Can you work these out from the model? Positions are in its coordinate system, mm. A direction names the side the tool comes from. Coordinates: 2 decimals unless noted, no trailing zeros. Order: outer loops, then holes, each group sorted by start corner. A loop starts at its lowest first (then second) coordinate and runs counter-clockwise, first axis right, second up. Notation, with made-up numbers: (-2, 42) -> (3, 42) arc R20 cw to (3, 51) -> close; hole circle Ø1 at (59.5, 17). An arc over 180 degrees is marked (long way). Answer in a Markdown table with one row per item. Add a question column.
1. Imagine slicing it at D-D on y = -6. Write out the boundary of the cut face in (x, z).
2. On a 3-axis mill with a long thin cutter (end or side, diameter ignored), from which of +Z, -Z, +X, -X, +Y, -Y can I reach the whole of each face in a straight line? I mean faces 1 (the face through (2, -2, 2.5)), 2 (the face through (-5, 0, 40)), 3 (the face through (0, 6, 5)). Say none if no direction works.
3. Imagine slicing it at A-A on y = 0. Write out the boundary of the cut face in (x, z).
4. Imagine slicing it at C-C on x = 0. Write out the boundary of the cut face in (y, z), plus the area to 3 significant figures.
5. We'd pull the mould along Y, two halves only. Please class faces 4 (the face through (-0.29, 2.23, 1.23)), 5 (the face through (5, 0, 40)), 6 (the face through (-3.746, 0.165, 21.512)): pulls with the +Y half, pulls with the -Y half, needs draft (parallel to the pull), parting line crosses it, or undercut.
6. Will these pins go through, and if not, where does the flat tip stop? pin 1 (2 mm diameter, centred on y = 7, z = 18.5, fed in from -X); pin 2 (2 mm diameter, centred on x = -2.5, z = 23, fed in from -Y); pin 3 (1.5 mm diameter, centred on y = -6, z = 10.5, fed in from -X).
7. Imagine slicing it at B-B on z = 17.5. Write out the boundary of the cut face in (x, y), plus the area to 3 significant figures.
8. If I drill on line 1 along X through (y, z) = (0, 10); line 2 along Y through (x, z) = (0, 1.25), over which ranges is the centre line in solid material (lowest first)? Write a range as [from, to].
from build123d import *
from build123d.topology import SkipClean

# Parameters (mm, degrees)
CROQUIS1_R              = 10
CROQUIS1_R_2            = 2.25
SALIENTE_EXTRUIR1_DEPTH = 5
SALIENTE_EXTRUIR2_DEPTH = 35
CROQUIS3_R              = 1.5
CORTAR_EXTRUIR1_DEPTH   = 20
CROQUIS4_R              = 3.75
CORTAR_EXTRUIR2_DEPTH   = 2.5
CORTAR_EXTRUIR4_START   = 49
CROQUIS6_R              = 3.75
CORTAR_EXTRUIR4_DEPTH   = 49


with BuildPart() as part:
    # Croquis1 → Saliente-Extruir1 (new body)
    with BuildSketch(Plane.XY):
        Circle(CROQUIS1_R)
        Circle(CROQUIS1_R_2, mode=Mode.SUBTRACT)
    extrude(amount=SALIENTE_EXTRUIR1_DEPTH)

    # Croquis2 → Saliente-Extruir2 (add)
    with SkipClean():  # the faces are left unmerged after this step: merging them gives an invalid solid
        with BuildSketch(Plane.XY.offset(5)):
            with BuildLine():
                Line((-2.5, -9.682458366), (-2.5, 9.682458366))
                ThreePointArc((-2.5, 9.682458366), (-10, 0), (-2.5, -9.682458366))
            make_face()
            with BuildLine():
                Line((2.5, -9.682458366), (2.5, 9.682458366))
                ThreePointArc((2.5, 9.682458366), (10, 0), (2.5, -9.682458366))
            make_face()
        extrude(amount=SALIENTE_EXTRUIR2_DEPTH)
    add(part.part.scale(1), mode=Mode.REPLACE)  # the faces are merged on a copy

    # Croquis3 → Cortar-Extruir1 (cut, symmetric)
    with BuildSketch(Plane.ZY.offset(-2.5)):
        with Locations((35, 0)):
            Circle(CROQUIS3_R)
    extrude(amount=CORTAR_EXTRUIR1_DEPTH, both=True, mode=Mode.SUBTRACT)

    # Croquis4 → Cortar-Extruir2 (cut)
    with BuildSketch(Plane.XY.offset(5)):
        Circle(CROQUIS4_R)
    extrude(amount=-CORTAR_EXTRUIR2_DEPTH, mode=Mode.SUBTRACT)

    # Croquis6 → Cortar-Extruir4 (cut)
    with SkipClean():  # the faces are left unmerged after this step: merging them gives an invalid solid
        with BuildSketch(Plane.XY.offset(2.5).offset(CORTAR_EXTRUIR4_START)):
            Circle(CROQUIS6_R)
        extrude(amount=-CORTAR_EXTRUIR4_DEPTH, mode=Mode.SUBTRACT)


solid = part.part
Answers follow:
| question | item | result |
|---|---|---|
| 1 | outline | (-8, 0) -> (8, 0) -> (8, 40) -> (2.5, 40) -> (2.5, 5) -> (-2.5, 5) -> (-2.5, 40) -> (-8, 40) -> close |
| 2 | face 1 | +Z |
| 2 | face 2 | +Z, +X, -X, +Y, -Y |
| 2 | face 3 | +Z, +Y, -Y |
| 3 | outline | (-10, 0) -> (-2.25, 0) -> (-2.25, 2.5) -> (-3.75, 2.5) -> (-3.75, 33.5) -> (-10, 33.5) -> close; (-10, 36.5) -> (-3.75, 36.5) -> (-3.75, 40) -> (-10, 40) -> close; (2.25, 0) -> (10, 0) -> (10, 33.5) -> (3.75, 33.5) -> (3.75, 2.5) -> (2.25, 2.5) -> close; (3.75, 36.5) -> (10, 36.5) -> (10, 40) -> (3.75, 40) -> close |
| 4 | outline | (-10, 0) -> (-2.25, 0) -> (-2.25, 2.5) -> (-3.75, 2.5) -> (-3.75, 5) -> (-10, 5) -> close; (2.25, 0) -> (10, 0) -> (10, 5) -> (3.75, 5) -> (3.75, 2.5) -> (2.25, 2.5) -> close |
| 4 | area | 70.0 mm² |
| 5 | face 4 | undercut |
| 5 | face 5 | needs draft |
| 5 | face 6 | undercut |
| 6 | pin 1 | stops at x = -8 |
| 6 | pin 2 | stops at y = -9.68 |
| 6 | pin 3 | stops at x = -8.51 |
| 7 | outline | (-2.5, -9.68) -> (-2.5, -2.8) arc R3.75 cw to (-2.5, 2.8) -> (-2.5, 9.68) arc R10 ccw to start; (2.5, -9.68) arc R10 ccw to (2.5, 9.68) -> (2.5, 2.8) arc R3.75 cw to (2.5, -2.8) -> close |
| 7 | area | 206 mm² |
| 8 | line 1 | x = [-10, -3.75], [3.75, 10] |
| 8 | line 2 | y = [-10, -2.25], [2.25, 10] |
